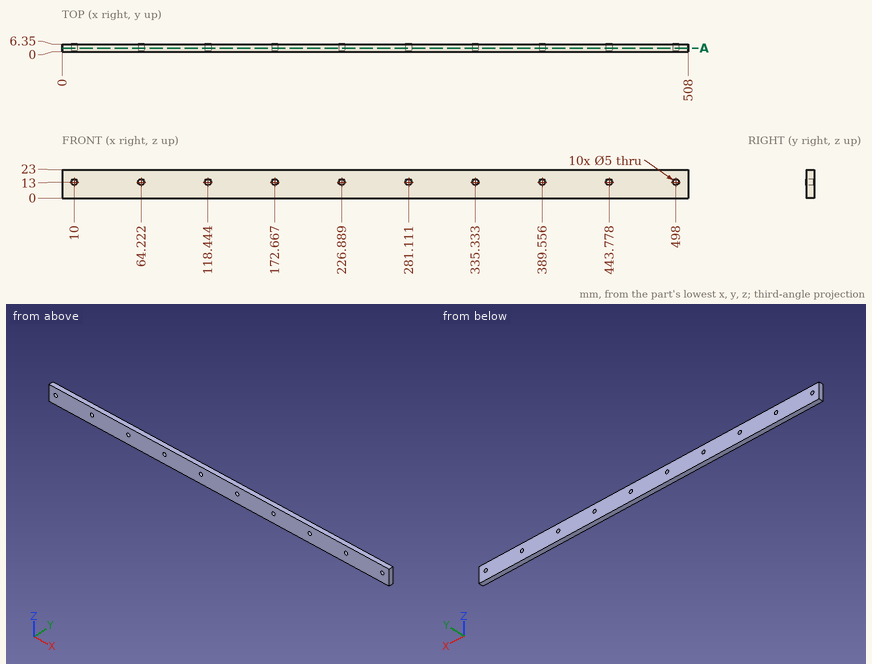
Study the drawing (mm; zero at the part's minimum x, y, z) and answer. Give positions to 0.01 mm unless a question says otherwise; leave off trailing zeros. Return JSON: item names as keys, results as strings. Group by question number.
1. Straight lines are drawn through the part: line 1 (Z direction, x = 65, y = 4) (1 decimal); line 2 (Z direction, x = 174, y = 4.75) (1 decimal). For each, find the intervals that lie inside material, in ascending order. Write a range as [from, to].
2. Find section A-A (y = 3). State how many separate pieces and enclosed holes the cut face has, then the cut area to 3 significant figures.
3. Given pin 1 Ø4.5 at (x, z) = (498, 13) entering from -Y, flat-ended and moving along its own axis, determine where the tip first touches the part or whether it passes through.
Verdict:
{
 "1": {"line 1": "z = [0, 10.6], [15.4, 23]", "line 2": "z = [0, 10.9], [15.1, 23]"},
 "2": {"separate pieces": "1", "enclosed holes": "10", "area": "11,500 mm^2"},
 "3": {"pin 1": "passes through"}
}
